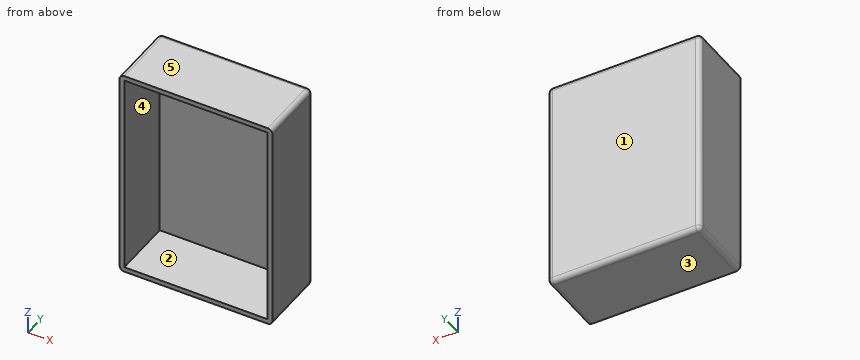
```python
from build123d import *

# Parameters (mm, degrees)
SKETCH1_W           = 95.4
SKETCH1_H           = 133.5
SKETCH1_W_2         = 89.4
SKETCH1_H_2         = 127.5
EXTRUDE_THIN1_DEPTH = 37.45
SKETCH2_W           = 95.4
SKETCH2_H           = 133.5
BOSS_EXTRUDE1_DEPTH = 5
FILLET3_R           = 3
FILLET4_R           = 3


with BuildPart() as part:
    # Sketch1 → Extrude-Thin1 (new body)
    with BuildSketch(Plane(origin=(0, 0, 0), x_dir=(1, 0, 0), z_dir=(0, 1, 0))):
        with Locations((-0.544500843, -0.326636011)):
            Rectangle(SKETCH1_W, SKETCH1_H)
        with Locations((-0.544500843, -0.326636011)):
            Rectangle(SKETCH1_W_2, SKETCH1_H_2, mode=Mode.SUBTRACT)
    extrude(amount=EXTRUDE_THIN1_DEPTH)

    # Sketch2 → Boss-Extrude1 (add)
    with BuildSketch(Plane(origin=(0, 37.45, 0), x_dir=(1, 0, 0), z_dir=(0, 1, 0))):
        with Locations((-0.544500843, -0.326636011)):
            Rectangle(SKETCH2_W, SKETCH2_H)
    extrude(amount=BOSS_EXTRUDE1_DEPTH)

    # Fillet3
    fillet3_edges = [part.edges().sort_by_distance(p)[0] for p in [
        (47.155499157, 21.225, 67.076636011),
        (-48.244500843, 21.225, 67.076636011),
        (-48.244500843, 21.225, -66.423363989),
        (47.155499157, 21.225, -66.423363989),
    ]]
    fillet(fillet3_edges, radius=FILLET3_R)

    # Fillet4
    fillet4_edges = [part.edges().sort_by_distance(p)[0] for p in [
        (-0.544500843, 42.45, 67.076636011),
        (-48.244500843, 42.45, 0.326636011),
        (47.155499157, 42.45, 0.326636011),
        (-0.544500843, 42.45, -66.423363989),
        (-47.365821187, 42.45, -65.544684332),
        (46.2768195, 42.45, -65.544684332),
        (46.2768195, 42.45, 66.197956355),
        (-47.365821187, 42.45, 66.197956355),
    ]]
    fillet(fillet4_edges, radius=FILLET4_R)


solid = part.part
```
Design review of the part built by this model. Coordinates are the model's own, in mm. Face numbers are marked on the shaded views. A direction names the side the tool comes from. Give positions to 0.01 mm unless a question says otherwise; leave off trailing zeros. Loops run counter-clockwise (first coordinate to the right, second up) from the corner with the lowest first, then second, coordinate; pieces in that order, holes last. Notation, with made-up numbers: (82.25, 76.5) -> (91.25, 76.5) arc R3 ccw to (91.25, 81.5) -> close; hole circle Ø6 at (-1, 81). An arc over 180 degrees is marked (long way). One line per item, written item: value.
Q1. We need section C-C on x = 38.5. Give the boundary of the cut face in (y, z), and give its area (3 significant figures).
Numbers:
outline: (0, -66.42) -> (39.45, -66.42) arc R3 ccw to (42.45, -63.42) -> (42.45, 64.08) arc R3 ccw to (39.45, 67.08) -> (0, 67.08) -> (0, 64.08) -> (37.45, 64.08) -> (37.45, -63.42) -> (0, -63.42) -> close
area: 888 mm^2
Q2. Machinability: for the marked faces 1 and 2, which of the approach directions +Z, -Z, +X, -X, +Y, -Y give a long, thin tool a straight path to every point of the face, cutting with its end or side? Answer none if there is none.
Numbers:
face 1: +Z, -Z, +X, -X, +Y
face 2: -Y
Q3. We need section A-A on y = 16. Give the boundary of the cut face in (x, z).
Numbers:
outline: (-48.24, -63.42) arc R3 ccw to (-45.24, -66.42) -> (44.16, -66.42) arc R3 ccw to (47.16, -63.42) -> (47.16, 64.08) arc R3 ccw to (44.16, 67.08) -> (-45.24, 67.08) arc R3 ccw to (-48.24, 64.08) -> close; hole (-45.24, -63.42) -> (44.16, -63.42) -> (44.16, 64.08) -> (-45.24, 64.08) -> close
Q4. Draft analysis for pull direction Z (two halves, no side actions). For the marked faces 3, 4 and 5, state which applies: pulls with the +Z half, pulls with the -Z half, needs draft (parallel to the pull), parting line crosses it, or undercut.
Numbers:
face 3: pulls with the -Z half
face 4: undercut
face 5: pulls with the +Z half
Q5. We need section B-B on z = -35.5. Give the boundary of the cut face in (x, y).
Numbers:
outline: (-48.24, 0) -> (-45.24, 0) -> (-45.24, 37.45) -> (44.16, 37.45) -> (44.16, 0) -> (47.16, 0) -> (47.16, 39.45) arc R3 ccw to (44.16, 42.45) -> (-45.24, 42.45) arc R3 ccw to (-48.24, 39.45) -> close
Q6. For pin 1 Ø8 at (x, z) = (-36, 48.5) entering from -Y, flat-tipped, find the tip position at first contact; note if it passes through.
Numbers:
pin 1: stops at y = 37.45
Q7. For L1, parallel to X at y = 21, z = 22; L2, parallel to Z at x = -31.5, y = 28.5; L3, parallel to Y at x = -11.5, z = 4, list the stretches that pass through material, from the lowest coordinate up.
Numbers:
L1: x = -48.24 to -45.24, 44.16 to 47.16
L2: z = -66.42 to -63.42, 64.08 to 67.08
L3: y = 37.45 to 42.45
